from build123d import *

# Parameters (mm, degrees)
ENL_V_MAT_EXTRU_1_DEPTH = 15


with BuildPart() as part:
    # Esquisse1 → Révolution1 (revolve)
    with BuildSketch(Plane.XY, mode=Mode.PRIVATE) as r_volution1_sk:
        Polygon((0, 0), (-60, 0), (-120, 60), (-128, 60), (-68, 0), (-68, -6), (-80, -6), (-80, -20), (0, -20), align=None)
    revolve(r_volution1_sk.sketch.rotate(Axis((0, -20, 0), (0, 1, 0)), 270), axis=Axis((0, -20, 0), (0, 1, 0)))  # turned: the seam where the file's is

    # Esquisse8 → Enlèv. mat.-Extru.1 (cut, through all)
    with BuildSketch(Plane(origin=(0, -6, 0), x_dir=(1, 0, 0), z_dir=(0, 1, 0))):
        Polygon((-79.781170075, 5.913112665), (-40.797993833, -68.815141497), (-98.313445601, -98.818987004), (-137.296621843, -24.090732842), align=None)
    extrude(amount=-ENL_V_MAT_EXTRU_1_DEPTH, mode=Mode.SUBTRACT)


solid = part.part
Verification items for the finished model (mm, model axes). A direction names the side the tool comes from. Give positions to 0.01 mm unless a question says otherwise; leave off trailing zeros. Order: outer loops, then holes, each group sorted by start corner. A loop starts at its lowest first (then second) coordinate and runs counter-clockwise, first axis right, second up. Notation, with made-up numbers: M 9,-13 L 54,-13 A30 cw 54,13 Z; hole C 42,-34.75 d9. An arc over 180 degrees is marked long. Answer as a JSON object with one key per item and string values. Group by question number.
1) Depth check by flat-ended pin: pin 1 Ø2 at (y, z) = (-11, -17.5) entering from +X; pin 2 Ø12 at (y, z) = (-1.5, -55) entering from -X; pin 3 Ø12 at (x, y) = (-87.5, 2) entering from +Z; pin 4 Ø1.5 at (y, z) = (2, 35.5) entering from +X. Enter the tip coordinate at first touch or a pass-through.
2) Access from +Z, -Z, +X, -X, +Y, -Y to the whole of each face (thin tool, end or side, straight path). Record for faces 1 (the face through (62.91, 2.91, -32.72)), 2 (the face through (37.3, 60, -114.4)), 3 (the face through (-1, -20, 1)), 4 (the face through (-1, 0, -1)), 5 (the face through (-60.56, -12.9, 30.93)).
3) Cross-section at A-A (x = 0). Enter the section's corners in (y, z), then the cut area to 3 significant figures.
4) Scan lines: line 1 along Y through (x, z) = (-17, 15.5); line 2 along Z through (x, y) = (70.5, 53); line 3 along X through (y, z) = (38, -68). Record each from-to range of solid material in increasing order. Write a range as [from, to].
5) Cross-section at C-C (z = 0). Enter the section's corners in (x, y), then the cut area to 3 significant figures.
6) Cross-section at B-B (y = 7.5). Enter the section's corners in (x, z), then the cut area to 3 significant figures.
7) Mould release check, pull along Z, two halves, no side actions. Record for faces 6 (the face through (72.22, -13.1, -34.41)), 7 (the face through (56.56, 3.753, -29.418)), 8 (the face through (65, -6, -24)): released by +Z, released by -Z, zero draft, split by the parting line, or undercut.
Result sheet:
{
 "1": {"pin 1": "stops at x = 78.28", "pin 2": "stops at x = -61.61", "pin 3": "passes through", "pin 4": "stops at x = 61.3"},
 "2": {"face 1": "none", "face 2": "+Z, -Z, +X, -X, +Y", "face 3": "+Z, -Z, +X, -X, -Y", "face 4": "+Y", "face 5": "+Z, -X, -Y"},
 "3": {"outline": "M -20,-80 L -6,-80 L -6,-68 L 0,-68 L 60,-128 L 60,-120 L 0,-60 L 0,60 L 60,120 L 60,128 L 0,68 L -6,68 L -6,80 L -20,80 Z", "area": "4,020 mm2"},
 "4": {"line 1": "y = [-20, 0]", "line 2": "z = [-98.34, -88.31], [88.31, 98.34]", "line 3": "x = [-81.31, -70.57], [70.57, 81.31]"},
 "5": {"outline": "M -128,60 L -68,0 L -68,-6 L -76.7,-6 L -76.7,-20 L 80,-20 L 80,-6 L 68,-6 L 68,0 L 128,60 L 120,60 L 60,0 L -60,0 L -120,60 Z", "area": "3,970 mm2"},
 "6": {"outline": "C 0,0 d151; hole C 0,0 d135", "area": "3,590 mm2"},
 "7": {"face 6": "split by the parting line", "face 7": "undercut", "face 8": "zero draft"}
}
